Check sheet for the drawn part. Datum: minimum x, y, z corner. Units: mm. Round coordinates to 2 decimals unless told otherwise and drop trailing zeros. Write each loop counter-clockwise with the first axis right and the second up, starting at its lowest first coordinate (ties: lowest second). Pieces come first, ordered by that corner, then holes. Notation, with made-up numbers: (-32.5, 47) -> (-6.5, 47) arc R27 cw to (-6.5, 73) -> close; hole circle Ø6 at (19.25, 29.25). An arc over 180 degrees is marked (long way). Use CSV: the item, a comma, the result in double quotes.
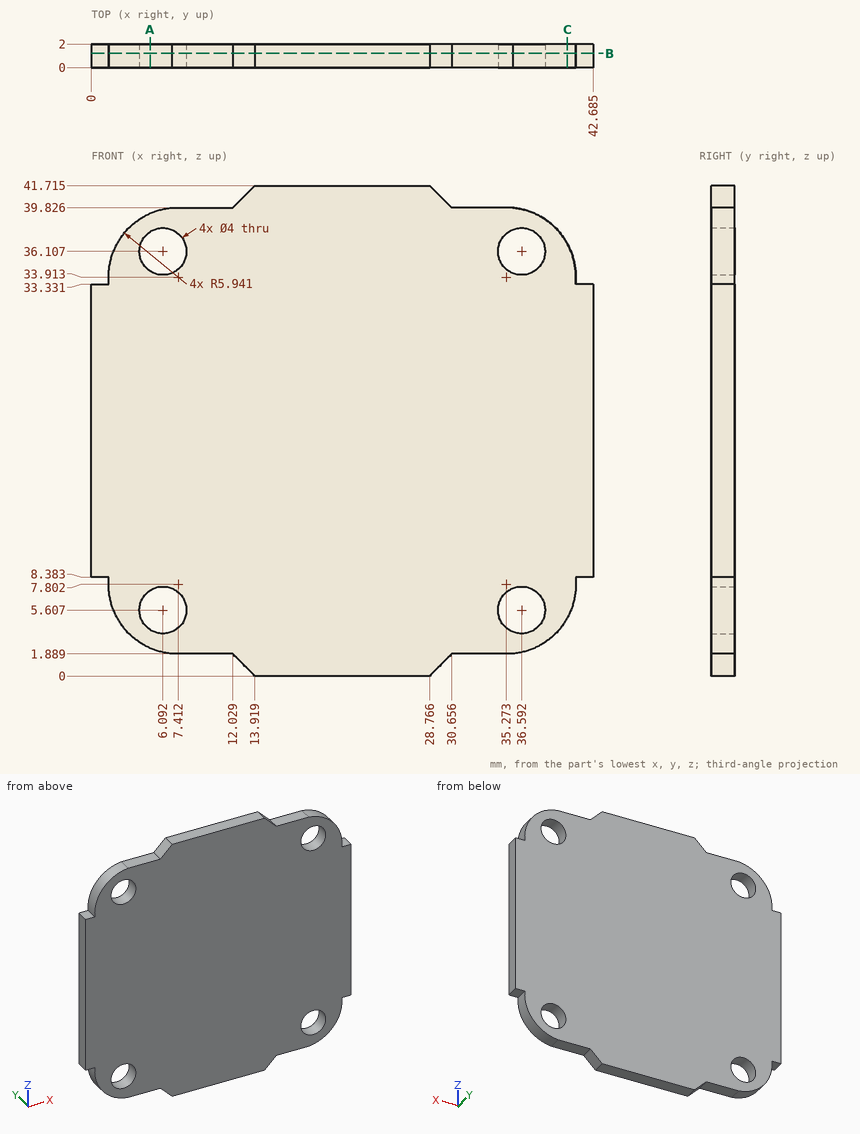
Q1. Material ranges on L1, parallel to Z at x = 5, y = 1.3; L2, parallel to X at y = 1.95, z = 35.5; L3, parallel to Z at x = 10.5, y = 1.1 (1 decimal), recorded low to high.
Filled in:
L1,"2.37 to 3.93, 7.28 to 34.43, 37.78 to 39.34"
L2,"1.69 to 4.19, 8 to 34.69, 38.5 to 41"
L3,"1.9 to 39.8"
Q2. Section check A-A (x = 5). Record the cut outline in (y, z).
Filled in:
outline,"(0, 2.37) -> (2, 2.37) -> (2, 3.93) -> (0, 3.93) -> close; (0, 7.28) -> (2, 7.28) -> (2, 34.43) -> (0, 34.43) -> close; (0, 37.78) -> (2, 37.78) -> (2, 39.34) -> (0, 39.34) -> close"
Q3. Section check B-B (y = 1.2). Record the cut outline in (x, z) (1 decimal), plus the area to 3 significant figures.
Filled in:
outline,"(0, 8.4) -> (1.5, 8.4) arc R5.9 ccw to (6.8, 1.9) -> (12, 1.9) -> (13.9, 0) -> (28.8, 0) -> (30.7, 1.9) -> (35.9, 1.9) arc R5.9 ccw to (41.2, 8.4) -> (42.7, 8.4) -> (42.7, 33.3) -> (41.2, 33.3) arc R5.9 ccw to (35.9, 39.8) -> (30.7, 39.8) -> (28.8, 41.7) -> (13.9, 41.7) -> (12, 39.8) -> (6.8, 39.8) arc R5.9 ccw to (1.5, 33.3) -> (0, 33.3) -> close; hole circle Ø4 at (6.1, 5.6); hole circle Ø4 at (6.1, 36.1); hole circle Ø4 at (36.6, 5.6); hole circle Ø4 at (36.6, 36.1)"
area,"1,560 mm²"
Q4. Section check C-C (x = 40.5). Record the cut outline in (y, z).
Filled in:
outline,"(0, 4.98) -> (2, 4.98) -> (2, 36.74) -> (0, 36.74) -> close"
Q5. Go/stop test with flat-tipped pins: P1, Ø0.6, axis at x = 8.5, y = 1, coming from the -Z side; P2, Ø0.6, axis at x = 34.5, y = 1, coming from the +Z side; P3, Ø1.2, axis at x = 42, y = 1, coming from the +Z side. Record where each tip stops, or that it passes through.
Filled in:
P1,"z = 1.89"
P2,"z = 39.83"
P3,"z = 33.33"
